Autodesk Inventor part; units mm, degrees
ref_plane "YZ Plane" through (0, 0, 0) normal (1, 0, 0) x (0, 1, 0)
ref_plane "XZ Plane" through (0, 0, 0) normal (0, 1, 0) x (-1, 0, 0)
ref_plane "XY Plane" through (0, 0, 0) normal (0, 0, 1) x (1, 0, 0)
sketch "Sketch1" plane through (0, 0, 0) normal (0, 1, 0) x (-1, 0, 0)
  line L0 (0, 0) -> (20, 0)
  line L1 (20, -30) -> (0, -30)
  line L2 (0, -30) -> (0, 0)
  line L3 (20, 0) -> (20, -10)
  line L4 (20, -10) -> (10, -10)
  line L5 (10, -10) -> (10, -20)
  line L6 (10, -20) -> (20, -20)
  line L7 (20, -20) -> (20, -30)
  dimension "d0" = 20
  dimension "d1" = 30
  dimension "d2" = 10
  dimension "d3" = 10
  dimension "d4" = 10
  dimension "d5" = 10
  dimension "d8" = 20
extrude "Extrusion1" add sketch "Sketch1" along normal blind 10
sketch "Sketch2" plane through (-20, 0, 0) normal (0, 0, 1) x (1, 0, 0)
  line L0 (0, 0) -> (0, 10)
  line L1 (0, 10) -> (20, 10)
  point P0 (20, 0)
  point P1 (5, 5)
  dimension "d16" = 5
  dimension "d17" = 5
hole "Hole1" at (-15, 5, 0) direction (0, 0, -1) diameter 1.5 depth 11 counterbore diameter 6.2 counterbore depth 9
sketch "Sketch3" plane through (0, 0, -30) normal (0, 0, -1) x (-1, 0, 0)
  line L0 (20, 0) -> (20, 10)
  line L1 (0, 10) -> (20, 10)
  point P0 (0, 0)
  point P1 (15, 5)
  dimension "d25" = 5
  dimension "d26" = 5
hole "Hole2" at (-15, 5, -30) direction (0, 0, 1) diameter 1.5 depth 11 counterbore diameter 6.2 counterbore depth 9
sketch "Sketch4" plane through (0, 0, 0) normal (1, 0, 0) x (0, 0, -1)
  line L0 (0, 10) -> (30, 10)
  line L1 (30, 0) -> (30, 10)
  point P0 (0, 0)
  point P1 (15, 5)
  dimension "d34" = 5
  dimension "d35" = 15
hole "Hole3" at (0, 5, -15) direction (-1, 0, 0) diameter 3.1 depth 20
fillet "Fillet1" radius 3.175 1 edges at (-10, 5, -20)
fillet "Fillet2" radius 3.175 1 edges at (-10, 5, -10)
fillet "Fillet3" radius 1.905 1 edges at (-20, 5, -20)
fillet "Fillet4" radius 1.905 1 edges at (-20, 5, -10)
fillet "Fillet5" radius 8.89 1 edges at (0, 5, -30)
fillet "Fillet6" radius 8.89 1 edges at (0, 5, 0)
properties part number "lickPort1"
The listing builds one solid part. Answer for the finished solid, in the listing's coordinates (mm). A direction names the side the tool comes from. Coordinates: 2 decimals unless noted, no trailing zeros. Write each loop counter-clockwise with the first axis right and the second up, starting at its lowest first coordinate (ties: lowest second). Pieces come first, ordered by that corner, then holes. Notation, with made-up numbers: (-11.5, -37.5) - (39.5, -37.5) arc R20 ccw to (39.5, -26.5) - close; hole circle Ø4 at (78.25, 62). An arc over 180 degrees is marked (long way). One line per item, written item: value.
1) Find section B-B (x = -15). Give the vertices of the cut face in (y, z).
Geometry check:
outline: (0, -30) - (1.9, -30) - (1.9, -21) - (4.25, -21) - (4.25, -20) - (0, -20) - close; (0, -10) - (4.25, -10) - (4.25, -9) - (1.9, -9) - (1.9, 0) - (0, 0) - close; (5.75, -21) - (8.1, -21) - (8.1, -30) - (10, -30) - (10, -20) - (5.75, -20) - close; (5.75, -10) - (10, -10) - (10, 0) - (8.1, 0) - (8.1, -9) - (5.75, -9) - close
2) Find section A-A (y = 5). Count the separate pieces of the cut face and the enclosed holes in it, and give its area (3 significant figures).
Geometry check:
separate pieces: 4
enclosed holes: 0
area: 323 mm2
3) Find section D-D (x = -11.25). Give the vertices of the cut face in (y, z), and give its area (3 significant figures).
Geometry check:
outline: (0, -30) - (10, -30) - (10, -19.35) - (0, -19.35) - close; (0, -10.65) - (10, -10.65) - (10, 0) - (0, 0) - close
area: 213 mm2
4) Each of these flat-tipped pins is pushed along its axis until it touches: pin 1 Ø2.5 at (y, z) = (5, -15) entering from -X; pin 2 Ø6 at (x, y) = (-11, 8) entering from +Z; pin 3 Ø5.5 at (x, y) = (-15, 5) entering from -Z; pin 4 Ø1 at (y, z) = (5.5, -25) entering from +X. Where does it stop, or does it pass through?
Geometry check:
pin 1: passes through
pin 2: stops at z = 0
pin 3: stops at z = -21
pin 4: stops at x = -0.67
5) For a pull along X with two mould halves and no side action, classify faces 6 (the cylindrical face through (-19.457, 5.07, -20.573)), 7 (the cylindrical face through (-15.51, 5.55, -9.51)), 8 (the flat face through (0, 3.8, -13.7)) as pulls with the +X half, pulls with the -X half, needs draft (parallel to the pull), parting line crosses it, or undercut.
Geometry check:
face 6: pulls with the -X half
face 7: undercut
face 8: pulls with the +X half
6) A tool of negligible diameter and unlimited length cuts with its end or side. For faces 1 (the flat face through (-14, 4, -9)), 2 (the flat face through (-14, 6, -21)), 3 (the flat face through (-12, 3, -30)), 4 (the flat face through (-8, 10, -15)), 5 (the flat face through (-16, 5, -20)), from which of +Z, -Z, +X, -X, +Y, -Y can it reach the whole face along a straight path? Write none if from no direction.
Geometry check:
face 1: +Z
face 2: -Z
face 3: -Z, +X, -X, +Y, -Y
face 4: +Z, -Z, +X, -X, +Y
face 5: -X, +Y, -Y
7) Find section C-C (z = -15). Give the vertices of the cut face in (x, y).
Geometry check:
outline: (-10, 0) - (0, 0) - (0, 3.45) - (-10, 3.45) - close; (-10, 6.55) - (0, 6.55) - (0, 10) - (-10, 10) - close
8) Consider line 1 along Y through (x, z) = (-15, -9.6); line 2 along Z through (x, y) = (-13.25, 8.75); line 3 along Z through (x, y) = (-4.25, 5). Determine where each line is inside the solid, lowest interval first. Write a range as from..to.
Geometry check:
line 1: y = 0..4.25, 5.75..10
line 2: z = -30..-20, -10..0
line 3: z = -28.69..-16.55, -13.45..-1.31
